Design review of the part built by this model. Coordinates are the model's own, in mm. Face numbers are marked on the shaded views. Coordinates: 2 decimals unless noted, no trailing zeros. Order: outer loops, then holes, each group sorted by start corner. A loop starts at its lowest first (then second) coordinate and runs counter-clockwise, first axis right, second up. Notation, with made-up numbers: M 24,37.25 L 37,37.25 A9 ccw 37,54.25 Z; hole C 20.25,3 d2. An arc over 180 degrees is marked long. Answer as a JSON object with one key per item and string values.
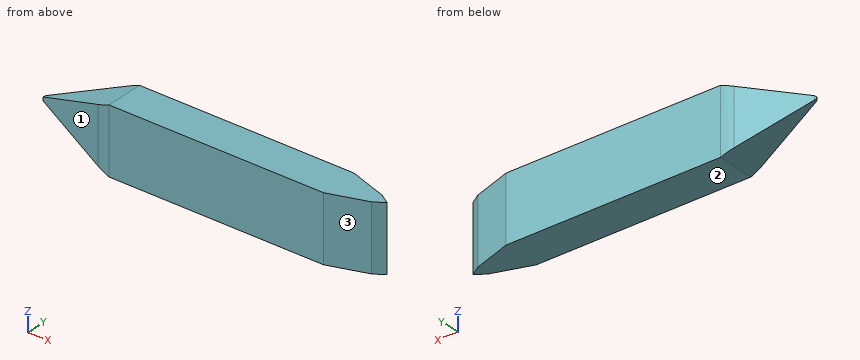
from build123d import *

# Parameters (mm, degrees)
F1_DEPTH = 25
F3_DEPTH = 14.524811


with BuildPart() as f1:
    # F0 (on Top) → F1 (new body)
    with BuildSketch(Plane.XY):
        with BuildLine():
            Line((56.428571, 2.5), (41.904763, 7.261906))
            Line((41.904763, 7.261906), (-39.518585, 7.261906))
            ThreePointArc((-39.518585, 7.261906), (-41.887959, 7.121061), (-44.223962, 6.700512))
            Line((-44.223962, 6.700512), (-69.89717, 0.485965))
            ThreePointArc((-69.89717, 0.485965), (-70.279535, 0), (-69.89717, -0.485965))
            Line((-69.89717, -0.485965), (-44.223962, -6.700512))
            ThreePointArc((-44.223962, -6.700512), (-41.887959, -7.121061), (-39.518585, -7.261906))
            Line((-39.518585, -7.261906), (41.904763, -7.261906))
            Line((41.904763, -7.261906), (56.428571, -2.5))
            Line((56.428571, -2.5), (60.23809, 0))
            Line((60.23809, 0), (56.428571, 2.5))
        make_face()
    extrude(amount=F1_DEPTH)

    # F2 (on face) → F3 (cut, through all)
    with BuildSketch(Plane.XZ.offset(7.261906)):
        with BuildLine():
            Line((-69.757227, 13.292665), (-39.518585, 25))
            Line((-39.518585, 25), (-72.551064, 25))
            Line((-72.551064, 25), (-72.551064, 0))
            Line((-72.551064, 0), (-39.518585, 0))
            Line((-39.518585, 0), (-69.757227, 11.707335))
            ThreePointArc((-69.757227, 11.707335), (-70.300335, 12.5), (-69.757227, 13.292665))
        make_face()
    extrude(amount=-F3_DEPTH, mode=Mode.SUBTRACT)


solid = f1.part
1) Mouldability with a two-part tool opening along X and no side actions: class the marked faces 1, 2 and 3 as released by +X, released by -X, zero draft, split by the parting line, or undercut.
Taken from the geometry:
{"face 1": "released by -X", "face 2": "zero draft", "face 3": "released by +X"}
2) To check wall thickness, follow L1, parallel to Z at x = -50, y = 4.5; L2, parallel to Y at x = -51.5, z = 12; L3, parallel to Y at x = -47, z = 11. State the ranges of each line that lie inside material, in increasing order.
Taken from the geometry:
{"L1": "z = 4.06 to 20.94", "L2": "y = -4.94 to 4.94", "L3": "y = -6.03 to 6.03"}
3) Add section C-C (x = 44). State the section outline as (y, z) points.
Taken from the geometry:
{"outline": "M -6.57,0 L 6.57,0 L 6.57,25 L -6.57,25 Z"}
4) Add section B-B (y = -5.25). State the section outline as (x, z) points.
Taken from the geometry:
{"outline": "M -50.22,4.14 L -39.52,0 L 48.04,0 L 48.04,25 L -39.52,25 L -50.22,20.86 Z"}
5) Add section A-A (z = 5.5). State the section outline as (x, y) points.
Taken from the geometry:
{"outline": "M -53.72,-4.4 L -44.22,-6.7 A20 ccw -39.52,-7.26 L 41.9,-7.26 L 56.43,-2.5 L 60.24,0 L 56.43,2.5 L 41.9,7.26 L -39.52,7.26 A20 ccw -44.22,6.7 L -53.72,4.4 Z"}
6) Add section D-D (z = 18). State the section outline as (x, y) points, and give its area (3 significant figures).
Taken from the geometry:
{"outline": "M -57.6,-3.46 L -44.22,-6.7 A20 ccw -39.52,-7.26 L 41.9,-7.26 L 56.43,-2.5 L 60.24,0 L 56.43,2.5 L 41.9,7.26 L -39.52,7.26 A20 ccw -44.22,6.7 L -57.6,3.46 Z", "area": "1,540 mm2"}
7) Insertion check: pin 1 Ø6 at (x, z) = (-53.5, 15) entering from +Y; pin 2 Ø4 at (x, z) = (-57, 12.5) entering from -Y; pin 3 Ø1 at (x, y) = (-42.5, 1.5) entering from -Z. Each pin has a flat end and moves straight along its axis. Give the tip position at first contact, or say it passes through.
Taken from the geometry:
{"pin 1": "stops at y = 5.18", "pin 2": "stops at y = -4.09", "pin 3": "stops at z = 0.96"}
